The listing builds one solid part. Answer for the finished solid, in the listing's coordinates (mm). A direction names the side the tool comes from. Round coordinates to 2 decimals unless told otherwise and drop trailing zeros. Loops run counter-clockwise (first coordinate to the right, second up) from the corner with the lowest first, then second, coordinate; pieces in that order, holes last. Notation, with made-up numbers: (-33.5, 86) - (-13.5, 86) arc R13 ccw to (-13.5, 109) - close; hole circle Ø10 at (34, 6). An arc over 180 degrees is marked (long way). Write item = value, one per line. Start each with the question number.
1) For a pull along Z with two mould halves and no side action, classify faces 6 (the flat face through (-12, -3, 4)), 7 (the cylindrical face through (7.246, -12.479, 2.235)), 8 (the flat face through (-14, 2, 0)), 9 (the flat face through (-14, 14, 2)) as released by +Z, released by -Z, zero draft, split by the parting line, or undercut.
2) A tool of negligible diameter and unlimited length cuts with its end or side. For faces 1 (the flat face through (11.4, 1, 2)), 2 (the flat face through (0, -13, -3)), 3 (the flat face through (14, 2, 0)), 4 (the cylindrical face through (-8.075, -12.479, -1.235)), 5 (the flat face through (-17.4, 0, 2)), from which of +Z, -Z, +X, -X, +Y, -Y can it reach the whole face along a straight path? Write none if from no direction.
3) Section A-A, the plane z = -1.25 is taken. Determine the outline of the cut face in (x, y) (3 decimals).
4) Section D-D, the plane z = 0.5 is taken. Determine the outline of the cut face in (x, y).
5) Section C-C, the plane x = -2 is taken. Determine the outline of the cut face in (y, z) (3 decimals), and give its area (3 significant figures).
6) Section B-B, the plane y = 12.75 is taken. Determine the outline of the cut face in (x, z), and give its area (3 significant figures).
7) Straight lines are drawn through the part: line 1 along X through (y, z) = (-3.5, 0.75); line 2 along Y through (x, z) = (13.7, 2.65); line 3 along Z through (x, y) = (15.5, 3.5). For each, find the intervals that lie inside material, in ascending order.
8) Given pin 1 Ø3 at (x, y) = (13.7, 11) entering from +Z; pin 2 Ø3 at (x, y) = (-13.5, 1) entering from -Z, each flat-ended and moving along its own axis, determine where each tip first touches the part or whether it passes through.
from build123d import *

# Parameters (mm, degrees)
SKETCH_1_W          = 6
SKETCH_1_H          = 25
SKETCH_1_H_2        = 3
SKETCH_1_W_2        = 22.8
EXTRUDE_1_DEPTH     = 4
SKETCH_3_R          = 1.1
CUT_EXTRUDE_2_DEPTH = 23.688322988
SKETCH_4_W          = 34.8
SKETCH_4_H          = 3
EXTRUDE_2_DEPTH     = 3
CUT_EXTRUDE_3_DEPTH = 31.720677076


with BuildPart() as part:
    # 草图1 → 凸台-拉伸1 (new body)
    with BuildSketch(Plane.XY):
        with Locations((-14.4, 1.5)):
            Rectangle(SKETCH_1_W, SKETCH_1_H)
        with Locations((-14.4, -12.5)):
            Rectangle(SKETCH_1_W, SKETCH_1_H_2)
        with Locations((0, -12.5)):
            Rectangle(SKETCH_1_W_2, SKETCH_1_H_2)
        with Locations((14.4, -12.5)):
            Rectangle(SKETCH_1_W, SKETCH_1_H_2)
        with Locations((14.4, 1.5)):
            Rectangle(SKETCH_1_W, SKETCH_1_H)
    extrude(amount=EXTRUDE_1_DEPTH)

    # 草图3 → 切除-拉伸2 (cut, through all)
    with BuildSketch(Plane(origin=(0, 0, 0), x_dir=(-1, 0, 0), z_dir=(0, 0, -1))):
        with Locations((-13.7, 11)):
            Circle(SKETCH_3_R)
        with Locations((13.7, 11)):
            Circle(SKETCH_3_R)
    extrude(amount=-CUT_EXTRUDE_2_DEPTH, mode=Mode.SUBTRACT)

    # 草图4 → 凸台-拉伸2 (add)
    with BuildSketch(Plane.XZ.offset(14)):
        with Locations((0, -1.5)):
            Rectangle(SKETCH_4_W, SKETCH_4_H)
    extrude(amount=-EXTRUDE_2_DEPTH)

    # 草图5 → 切除-拉伸3 (cut, through all)
    with BuildSketch(Plane(origin=(0, -11, 0), x_dir=(1, 0, 0), z_dir=(0, 1, 0))):
        with BuildLine():
            Line((6.571482936, 0.575), (-7.4, 0.575))
            ThreePointArc((-7.4, 0.575), (-8.075, 1.25), (-7.4, 1.925))
            Line((-7.4, 1.925), (6.571482936, 1.925))
            ThreePointArc((6.571482936, 1.925), (7.246482936, 1.25), (6.571482936, 0.575))
        make_face()
        with BuildLine():
            Line((-7.4, -1.575), (6.571482936, -1.575))
            ThreePointArc((6.571482936, -1.575), (7.246482936, -2.25), (6.571482936, -2.925))
            Line((6.571482936, -2.925), (-7.4, -2.925))
            ThreePointArc((-7.4, -2.925), (-8.075, -2.25), (-7.4, -1.575))
        make_face()
    extrude(amount=-CUT_EXTRUDE_3_DEPTH, mode=Mode.SUBTRACT)


solid = part.part
Geometry check:
q1.face_6 = released by +Z
q1.face_7 = undercut
q1.face_8 = released by -Z
q1.face_9 = zero draft
q2.face_1 = +Z, -Z, +Y
q2.face_2 = -Z, +X, -X, +Y, -Y
q2.face_3 = -Z, +X, -X, +Y
q2.face_4 = +Y, -Y
q2.face_5 = +Z, -Z, -X, +Y, -Y
q3.outline = (-17.4, -14) - (-8.075, -14) - (-8.075, -11) - (-17.4, -11) - close; (7.246, -14) - (17.4, -14) - (17.4, -11) - (7.246, -11) - close
q4.outline = (-17.4, -14) - (17.4, -14) - (17.4, 14) - (11.4, 14) - (11.4, -11) - (-11.4, -11) - (-11.4, 14) - (-17.4, 14) - close; hole circle Ø2.2 at (-13.7, 11); hole circle Ø2.2 at (13.7, 11)
q5.outline = (-14, -3) - (-11, -3) - (-11, -1.925) - (-14, -1.925) - close; (-14, -0.575) - (-11, -0.575) - (-11, 1.575) - (-14, 1.575) - close; (-14, 2.925) - (-11, 2.925) - (-11, 4) - (-14, 4) - close
q5.area = 12.9 mm2
q6.outline = (-17.4, 0) - (-11.4, 0) - (-11.4, 4) - (-17.4, 4) - close; (11.4, 0) - (17.4, 0) - (17.4, 4) - (11.4, 4) - close
q6.area = 48.0 mm2
q7.line_1 = -17.4 to -11.4, 11.4 to 17.4
q7.line_2 = -14 to 9.9, 12.1 to 14
q7.line_3 = 0 to 4
q8.pin_1 = 4
q8.pin_2 = 0
